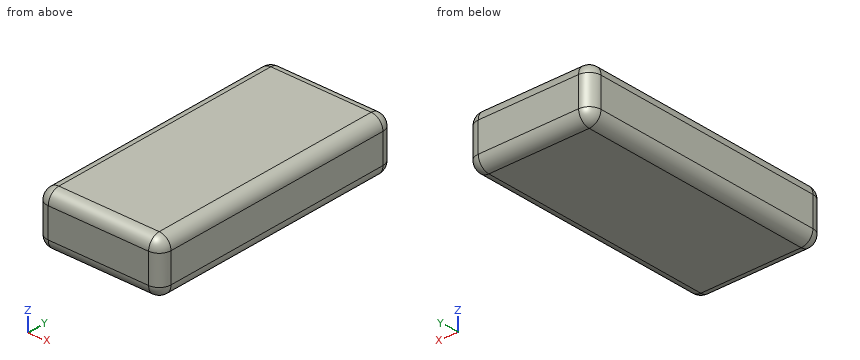
Autodesk Fusion 360 part; units mm, degrees
sketch "Sketch2" plane through (0, 0, 0) normal (0, 1, 0) x (1, 0, 0)
  line L0 (8.5, 4.5) -> (-8.5, 4.5)
  line L1 (-10.5, 2.5) -> (-10.5, -2.5)
  line L2 (-8.5, -4.5) -> (8.5, -4.5)
  line L3 (10.5, -2.5) -> (10.5, 2.5)
  line L4 (10.5, 4.5) -> (-10.5, -4.5) construction
  line L5 (-10.5, 4.5) -> (10.5, -4.5) construction
  arc A0 (-10.5, -2.5) -> (-8.5, -4.5) centre (-8.5, -2.5) ccw
  arc A1 (-8.5, 4.5) -> (-10.5, 2.5) centre (-8.5, 2.5) ccw
  arc A2 (10.5, 2.5) -> (8.5, 4.5) centre (8.5, 2.5) ccw
  arc A3 (8.5, -4.5) -> (10.5, -2.5) centre (8.5, -2.5) ccw
  dimension "d1" = 21
  dimension "d2" = 9
  dimension "d3" = 2
  dimension "d4" = 2
  dimension "d5" = 2
  dimension "d6" = 2
extrude "Extrude1" add sketch "Sketch2" along normal blind 44
fillet "Fillet1" radius 2 1 faces at (-2.8333, 0, -1.5)
fillet "Fillet2" radius 2 1 faces at (-2.8333, 44, -1.5)
Source: CAD feature listing. Evaluate the final solid. Frame: model axes, mm. Round coordinates to 2 decimals unless told otherwise and drop trailing zeros. Order: outer loops, then holes, each group sorted by start corner. A loop starts at its lowest first (then second) coordinate and runs counter-clockwise, first axis right, second up. Notation, with made-up numbers: (-28.75, 83) -> (7.25, 83) arc R26 cw to (7.25, 97) -> close; hole circle Ø8 at (59.25, 40). An arc over 180 degrees is marked (long way). Answer as CSV lines item,"result".
Item 1: Section A-A, the plane y = 8. Return loops of the section in (x, z), plus the area to 3 significant figures.
A:
outline,"(-10.5, -2.5) arc R2 ccw to (-8.5, -4.5) -> (8.5, -4.5) arc R2 ccw to (10.5, -2.5) -> (10.5, 2.5) arc R2 ccw to (8.5, 4.5) -> (-8.5, 4.5) arc R2 ccw to (-10.5, 2.5) -> close"
area,"186 mm²"
Item 2: Section B-B, the plane x = 9.25. Return loops of the section in (y, z).
A:
outline,"(0.15, -2.5) arc R1.85 ccw to (2, -4.35) -> (42, -4.35) arc R1.85 ccw to (43.85, -2.5) -> (43.85, 2.5) arc R1.85 ccw to (42, 4.35) -> (2, 4.35) arc R1.85 ccw to (0.15, 2.5) -> close"
Item 3: Line query: L1, parallel to Z at x = -9, y = 7; L2, parallel to X at y = 23.5, z = 3.75; L3, parallel to Y at x = 9.5, z = -1.75. Output: solid intervals per line, ascending.
A:
L1,"-4.44 to 4.44"
L2,"-10.06 to 10.06"
L3,"0.27 to 43.73"
Item 4: Pin query (flat end, axial travel): pin 1 Ø1.5 at (x, z) = (0, 2) entering from -Y; pin 2 Ø1.5 at (x, z) = (-2.5, -3.5) entering from +Y. Return the tip coordinate at first contact, or that it passes through.
A:
pin 1,"y = 0"
pin 2,"y = 43.98"
